from build123d import *

# Parameters (mm, degrees)
BOSS_EXTRUDE1_DEPTH = 400


with BuildPart() as part:
    # Sketch1 → Boss-Extrude1 (new, symmetric)
    with BuildSketch(Plane(origin=(0, 0, 0), x_dir=(0, 0, -1), z_dir=(1, 0, 0))):
        with BuildLine():
            Line((-15, 10), (15, 10))
            ThreePointArc((15, 10), (18.535533906, 8.535533906), (20, 5))
            Line((20, 5), (20, -5))
            ThreePointArc((20, -5), (18.535533906, -8.535533906), (15, -10))
            Line((15, -10), (-15, -10))
            ThreePointArc((-15, -10), (-18.535533906, -8.535533906), (-20, -5))
            Line((-20, -5), (-20, 5))
            ThreePointArc((-20, 5), (-18.535533906, 8.535533906), (-15, 10))
        make_face()
        with BuildLine():
            Line((12.148766077, 4.049588692), (12.148766077, -4.049588692))
            ThreePointArc((12.148766077, -4.049588692), (10.577040219, -4.75760445), (8.870332019, -5))
            Line((8.870332019, -5), (-8.870332019, -5))
            ThreePointArc((-8.870332019, -5), (-10.577040219, -4.75760445), (-12.148766077, -4.049588692))
            Line((-12.148766077, -4.049588692), (-12.148766077, 4.049588692))
            ThreePointArc((-12.148766077, 4.049588692), (-10.577040219, 4.75760445), (-8.870332019, 5))
            Line((-8.870332019, 5), (8.870332019, 5))
            ThreePointArc((8.870332019, 5), (10.577040219, 4.75760445), (12.148766077, 4.049588692))
        make_face(mode=Mode.SUBTRACT)
    extrude(amount=BOSS_EXTRUDE1_DEPTH, both=True)


solid = part.part
Work out the finished part from the listing and answer in its coordinate system (mm). A direction names the side the tool comes from. Coordinates: 2 decimals unless noted, no trailing zeros. Write each loop counter-clockwise with the first axis right and the second up, starting at its lowest first coordinate (ties: lowest second). Pieces come first, ordered by that corner, then holes. Notation, with made-up numbers: M -26,3 L -15,3 A20 cw -15,7 Z; hole C 58,-25 d9. An arc over 180 degrees is marked long. Use one line per item in the form item = value. Start each with the question number.
1. The mould has two halves that part along Z. Classify faces 1 (the face through (-400, -7, 0)), 2 (the face through (6, -5, 0)): released by +Z, released by -Z, zero draft, split by the parting line, or undercut.
2. The part is cut by section C-C (y = 0.75). Give the vertices of the cut face in (x, z), plus the area to 3 significant figures.
3. The part is cut by section A-A (z = -2.5). Give the vertices of the cut face in (x, y).
4. A tool of negligible diameter and unlimited length cuts with its end or side. For faces 3 (the face through (6, -10, 0)), 4 (the face through (6, 5, 0)), from which of +Z, -Z, +X, -X, +Y, -Y can it reach the whole face along a straight path? Write none if from no direction.
5. The part is cut by section B-B (x = 228.5). Give the vertices of the cut face in (y, z), plus the area to 3 significant figures.
6. Straight lines are drawn through the part: probe 1 along Z at (x, y) = (94, -0.25); probe 2 along Z at (x, y) = (31, -5.25); probe 3 along Y at (x, z) = (-342.5, 9.5). For each, find the intervals that lie inside material, in ascending order. Write a range as from..to.
Evaluation:
q1.face_1 = zero draft
q1.face_2 = undercut
q2.outline = M -400,-20 L 400,-20 L 400,-12.15 L -400,-12.15 Z; M -400,12.15 L 400,12.15 L 400,20 L -400,20 Z
q2.area = 12,600 mm^2
q3.outline = M -400,-10 L 400,-10 L 400,-5 L -400,-5 Z; M -400,5 L 400,5 L 400,10 L -400,10 Z
q4.face_3 = +Z, -Z, +X, -X, -Y
q4.face_4 = +X, -X
q5.outline = M -10,-15 A5 ccw -5,-20 L 5,-20 A5 ccw 10,-15 L 10,15 A5 ccw 5,20 L -5,20 A5 ccw -10,15 Z; hole M -5,-8.87 A6.13 ccw -4.05,-12.15 L 4.05,-12.15 A6.13 ccw 5,-8.87 L 5,8.87 A6.13 ccw 4.05,12.15 L -4.05,12.15 A6.13 ccw -5,8.87 Z
q5.area = 540 mm^2
q6.probe_1 = -20..-12.15, 12.15..20
q6.probe_2 = -19.99..19.99
q6.probe_3 = -10..-4.97, 4.97..10
